```python
from build123d import *

# Parameters (mm, degrees)
SKIZZE1_R                       = 13
AUFSATZ_LINEAR_AUSTRAGEN1_DEPTH = 2.5
SKIZZE2_R                       = 1.6
SCHNITT_LINEAR_AUSTRAGEN1_DEPTH = 102.387999648
FASE1_SIZE                      = 1.35
SKIZZE3_R                       = 1.85
SCHNITT_LINEAR_AUSTRAGEN2_DEPTH = 102.387999648


with BuildPart() as part:
    # Skizze1 → Aufsatz-Linear austragen1 (new body)
    # profile 1 of 2: a face of its own
    with BuildSketch(Plane(origin=(0, 0, 0), x_dir=(1, 0, 0), z_dir=(0, 1, 0))):
        with BuildLine():
            add(Edge.make_bspline(
                [(60.189363801, -0.001348653), (60.189363801, -17.15173776), (28.970752729, -44.530261837)],
                knots=[0, 0, 0, 1, 1, 1], degree=2))
            Line((28.970752729, -44.530261837), (28.970752729, -44.526849746))
            ThreePointArc((28.970752729, -44.526849746), (-79.200181402, 0.000357393), (28.970752729, 44.527564532))
            add(Edge.make_bspline(
                [(60.189363801, -0.001348653), (60.189363801, 17.149040455), (28.970752729, 44.527564532)],
                knots=[0, 0, 0, 1, 1, 1], degree=2))
        make_face()
        with Locations((47.189363801, -0.001348653)):
            Circle(SKIZZE1_R, mode=Mode.SUBTRACT)
    # profile 2 of 2: a face of its own
    with BuildSketch(Plane(origin=(0, 0, 0), x_dir=(1, 0, 0), z_dir=(0, 1, 0))):
        with Locations((47.189363801, -0.001348653)):
            Circle(SKIZZE1_R)
    extrude(amount=AUFSATZ_LINEAR_AUSTRAGEN1_DEPTH)

    # Skizze2 → Schnitt-Linear austragen1 (cut, through all)
    with BuildSketch(Plane(origin=(0, 2.5, 0), x_dir=(1, 0, 0), z_dir=(0, 1, 0))):
        with Locations(Location((51.189363801, 6.926854578, 0), (0, 0, 270))):
            Circle(SKIZZE2_R)
        with Locations(Location((51.189363801, -6.929551883, 0), (0, 0, 270))):
            Circle(SKIZZE2_R)
        with Locations(Location((39.189363801, -0.001348653, 0), (0, 0, 270))):
            Circle(SKIZZE2_R)
    extrude(amount=-SCHNITT_LINEAR_AUSTRAGEN1_DEPTH, mode=Mode.SUBTRACT)

    # Fase1
    fase1_edges = [part.edges().sort_by_distance(p)[0] for p in [
        (51.189363801, 2.5, -8.526854578),
        (51.189363801, 2.5, 5.329551883),
        (39.189363801, 2.5, -1.598651347),
    ]]
    chamfer(fase1_edges, length=FASE1_SIZE)

    # Skizze3 → Schnitt-Linear austragen2 (cut, through all)
    with BuildSketch(Plane(origin=(0, 2.5, 0), x_dir=(1, 0, 0), z_dir=(0, 1, 0))):
        with Locations(Location((-20.310636199, 33.998651347, 0), (0, 0, 270))):
            Circle(SKIZZE3_R)
        with Locations(Location((-20.310636199, -34.001348653, 0), (0, 0, 270))):
            Circle(SKIZZE3_R)
    extrude(amount=-SCHNITT_LINEAR_AUSTRAGEN2_DEPTH, mode=Mode.SUBTRACT)


solid = part.part
```
The model under review builds one solid part; all positions refer to its coordinate system, in mm. Round coordinates to 2 decimals unless told otherwise and drop trailing zeros. Order: outer loops, then holes, each group sorted by start corner. A loop starts at its lowest first (then second) coordinate and runs counter-clockwise, first axis right, second up. Notation, with made-up numbers: (-24, 76) -> (11, 76) arc R22 cw to (11, 101) -> close; hole circle Ø11 at (4.25, -26). An arc over 180 degrees is marked (long way). One line per item, written item: value. Start each with the question number.
Q1. Wall thickness on line 1 (X direction, y = 1.6, z = 6.5); line 2 (Z direction, x = 53.5, y = 2.35); line 3 (Z direction, x = 29, y = 1.85): over which ranges is each line inside the solid? List them lowest first.
Q2. Mouldability with a two-part tool opening along Z and no side actions: class faces 1 (the face through (-79.166, 1.232, 2.09)), 2 (the face through (40.54, 0.58, 0.86)), 3 (the face through (-10, 0, -1)) as released by +Z, released by -Z, zero draft, split by the parting line, or undercut.
Q3. Take a section at C-C (x = -42). Write out the cut boundary in (y, z).
Q4. Take a section at B-B (z = -47). Write out the cut boundary in (x, y).
Q5. Take a section at A-A (y = 1.7). Count the separate pieces of the cut face and the enclosed holes in it, and give its area (3 significant figures).
Reported:
1. line 1: x = -78.87 to 49.18, 53.19 to 59.18
1. line 2: z = -18.07 to -8.51, -5.35 to 5.35, 8.51 to 18.07
1. line 3: z = -44.5 to 44.5
2. face 1: split by the parting line
2. face 2: undercut
2. face 3: zero draft
3. outline: (0, -57.64) -> (2.5, -57.64) -> (2.5, 57.64) -> (0, 57.64) -> close
4. outline: (-58.28, 0) -> (26.38, 0) -> (26.38, 2.5) -> (-58.28, 2.5) -> close
5. separate pieces: 1
5. enclosed holes: 5
5. area: 13,100 mm2
